The model under review builds one solid part; all positions refer to its coordinate system, in mm. Face numbers are marked on the shaded views. A direction names the side the tool comes from. Round coordinates to 2 decimals unless told otherwise and drop trailing zeros. Write each loop counter-clockwise with the first axis right and the second up, starting at its lowest first coordinate (ties: lowest second). Pieces come first, ordered by that corner, then holes. Notation, with made-up numbers: M 43.25,-8 L 90.25,-8 A32 ccw 90.25,24 Z; hole C 18,74 d9. An arc over 180 degrees is marked long. One line per item, written item: value. Start each with the question number.
1) Tool access review of the marked faces 4 and 5: name each direction out of +Z, -Z, +X, -X, +Y, -Y from which nothing blocks a thin tool from reaching the whole face with its end or side.
2) Wall thickness on probe 1 along X at (y, z) = (0.5, -84); probe 2 along Z at (x, y) = (161.5, 2.25): over which ranges is each line inside the solid? List them lowest first.
3) Take a section at B-B, the plane z = -69. Write out the cut boundary in (x, y) (3 decimals).
4) Mouldability with a two-part tool opening along Z and no side actions: class the marked faces 1, 2 and 3 as +Z half, -Z half, draft (parallel to the pull), parting line (faces both ways), or undercut.
5) For P1, Ø4, axis at x = 125.5, z = -47, coming from the +Y side, flat-tipped, find the tip position at first contact; note if it passes through.
from build123d import *

# Parameters (mm, degrees)
SKETCH11_W     = 187.05178758
SKETCH11_H     = 103.91050065
EXTRUDE5_DEPTH = 18.923
SKETCH14_W     = 187.05178758
SKETCH14_H     = 103.91050065
EXTRUDE6_DEPTH = 3.175


with BuildPart() as part:
    # Sketch11 → Extrude5 (new body)
    with BuildSketch(Plane(origin=(0, 0, 0), x_dir=(1, 0, 0), z_dir=(0, 1, 0))):
        with Locations((93.52589379, 51.955250325)):
            Rectangle(SKETCH11_W, SKETCH11_H)
        with BuildLine():
            Line((9.525, 6.35), (116.541319734, 6.35))
            ThreePointArc((116.541319734, 6.35), (118.786383764, 7.27993597), (119.716319734, 9.525))
            Line((119.716319734, 9.525), (119.716319734, 24.585352544))
            Line((119.716319734, 24.585352544), (126.066319734, 24.585352544))
            Line((126.066319734, 24.585352544), (126.066319734, 9.525))
            ThreePointArc((126.066319734, 9.525), (126.996255703, 7.27993597), (129.241319734, 6.35))
            Line((129.241319734, 6.35), (177.52678758, 6.35))
            ThreePointArc((177.52678758, 6.35), (179.77185161, 7.27993597), (180.70178758, 9.525))
            Line((180.70178758, 9.525), (180.70178758, 94.38550065))
            ThreePointArc((180.70178758, 94.38550065), (179.77185161, 96.63056468), (177.52678758, 97.56050065))
            Line((177.52678758, 97.56050065), (129.241319734, 97.56050065))
            ThreePointArc((129.241319734, 97.56050065), (126.996255703, 96.63056468), (126.066319734, 94.38550065))
            Line((126.066319734, 94.38550065), (126.066319734, 79.325148105))
            Line((126.066319734, 79.325148105), (119.716319734, 79.325148105))
            Line((119.716319734, 79.325148105), (119.716319734, 94.38550065))
            ThreePointArc((119.716319734, 94.38550065), (118.786383764, 96.63056468), (116.541319734, 97.56050065))
            Line((116.541319734, 97.56050065), (9.525, 97.56050065))
            ThreePointArc((9.525, 97.56050065), (7.27993597, 96.63056468), (6.35, 94.38550065))
            Line((6.35, 94.38550065), (6.35, 9.525))
            ThreePointArc((6.35, 9.525), (7.27993597, 7.27993597), (9.525, 6.35))
        make_face(mode=Mode.SUBTRACT)
    extrude(amount=EXTRUDE5_DEPTH)

    # Sketch14 → Extrude6 (add)
    with BuildSketch(Plane(origin=(0, 0, 0), x_dir=(1, 0, 0), z_dir=(0, 1, 0))):
        with Locations((93.52589379, 51.955250325)):
            Rectangle(SKETCH14_W, SKETCH14_H)
    extrude(amount=-EXTRUDE6_DEPTH)


solid = part.part
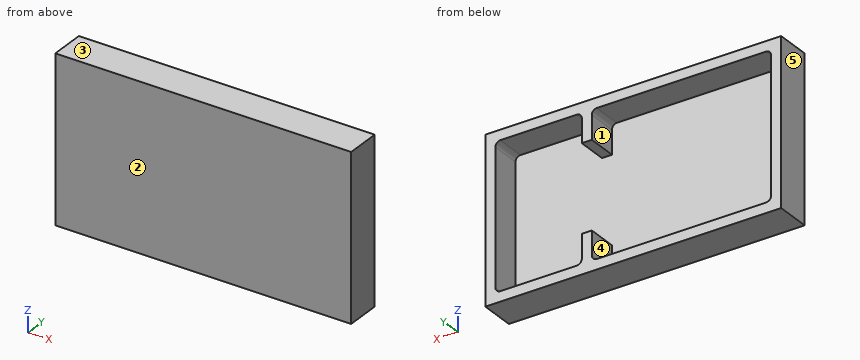
Checked values:
1. face 4: +Y
1. face 5: +Z, -Z, -X, +Y, -Y
2. probe 1: x = 0 to 6.35, 119.72 to 126.07, 180.7 to 187.05
2. probe 2: z = -103.91 to -97.56, -6.35 to 0
3. outline: M 0,-3.175 L 187.052,-3.175 L 187.052,18.923 L 180.702,18.923 L 180.702,0 L 6.35,0 L 6.35,18.923 L 0,18.923 Z
4. face 1: undercut
4. face 2: draft
4. face 3: +Z half
5. P1: stops at y = 0
